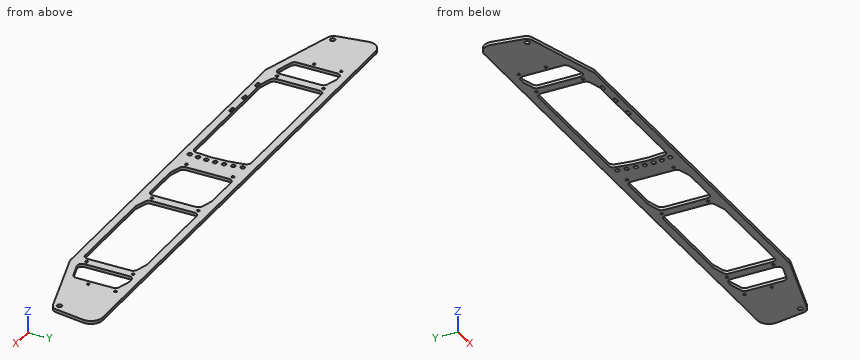
from build123d import *

# Parameters (mm, degrees)
SKETCH_1_R          = 3.25
EXTRUDE_1_DEPTH     = 4
HOLE_WIZARD_M52_D   = 5.5
HOLE_WIZARD_M53_D   = 5.5
FILLET_5_R          = 10
CUT_EXTRUDE_4_DEPTH = 354.032576401
FILLET_7_R          = 6
HOLE_WIZARD_M34_D   = 3.4
CUT_EXTRUDE_5_DEPTH = 354.032576401


with BuildPart() as part:
    # Эскиз1 → Бобышка-Вытянуть1 (new body)
    with BuildSketch(Plane.XY):
        with BuildLine():
            Line((-349.818316726, 28.672449915), (-342.910885265, -15.303620822))
            Line((-342.910885265, -15.303620822), (-240, -46))
            Line((-240, -46), (240, -46))
            Line((240, -46), (342.910885265, -15.303620822))
            Line((342.910885265, -15.303620822), (349.818316726, 28.672449915))
            ThreePointArc((349.818316726, 28.672449915), (346.399852001, 40.749019149), (335, 46))
            Line((335, 46), (-335, 46))
            ThreePointArc((-335, 46), (-346.399852001, 40.749019149), (-349.818316726, 28.672449915))
        make_face()
        with Locations((-335, -9.635315981)):
            Circle(SKETCH_1_R, mode=Mode.SUBTRACT)
        with Locations(Location((335, -9.635315981, 0), (0, 0, 180))):
            Circle(SKETCH_1_R, mode=Mode.SUBTRACT)
    extrude(amount=EXTRUDE_1_DEPTH)

    # Отверстие с зазором M52 (through all)
    with Locations(Plane(origin=(0, 0, 0), x_dir=(-1, 0, 0), z_dir=(0, 0, -1))):
        with Locations((215, -7)):
            Hole(HOLE_WIZARD_M52_D / 2)

    # Отверстие с зазором M53 (through all)
    with Locations(Plane(origin=(0, 0, 0), x_dir=(-1, 0, 0), z_dir=(0, 0, -1))):
        with Locations((31.771314746, 9.83), (35.189476411, 32.040691677), (33.141482074, 20.990703059), (31.085819286, -1.380913569), (31.085819286, -12.619086431), (31.771893326, -23.836297834), (33.141482074, -34.990703059)):
            Hole(HOLE_WIZARD_M53_D / 2)

    # Скругление5
    fillet_5_edges = [part.edges().sort_by_distance(p)[0] for p in [
        (342.910885265, -15.303620822, 2),
        (240, -46, 2),
        (-240, -46, 2),
        (-342.910885265, -15.303620822, 2),
    ]]
    fillet(fillet_5_edges, radius=FILLET_5_R)

    # Эскиз22 → Вырез-Вытянуть4 (cut, through all)
    with BuildSketch(Plane(origin=(0, 0, 0), x_dir=(-1, 0, 0), z_dir=(0, 0, -1))):
        Polygon((-227.540368898, -36), (-98.70593747, -36), (-79.540368898, -30.283271798), (-79.540368898, 36), (-208.374800326, 36), (-227.540368898, 30.283271798), align=None)
        with BuildLine():
            Line((227.54, -30.283271798), (208.374431428, -36))
            Line((208.374431428, -36), (40.898736363, -36))
            ThreePointArc((40.898736363, -36), (38.644905491, 0.150569256), (43.818079226, 36))
            Line((43.818079226, 36), (227.54, 36))
            Line((227.54, 36), (227.54, -30.283271798))
        make_face()
        Polygon((-271, 30.283271798), (-251.834431428, 36), (-239.540368898, 36), (-239.540368898, -35.701718831), (-271, -26.317903284), align=None)
        Polygon((-67.540368898, -36), (-13.70593747, -36), (5.459631102, -30.283271798), (5.459631102, 36), (-48.374800326, 36), (-67.540368898, 30.283271798), align=None)
        Polygon((239.54, 30.283271798), (258.705568572, 36), (271, 36), (271, -26.317903284), (239.54, -35.701828866), align=None)
    extrude(amount=-CUT_EXTRUDE_4_DEPTH, mode=Mode.SUBTRACT)

    # Скругление7
    fillet_7_edges = [part.edges().sort_by_distance(p)[0] for p in [
        (227.540368898, -36, 2),
        (227.540368898, 30.283271798, 2),
        (208.374800326, 36, 2),
        (79.540368898, 36, 2),
        (79.540368898, -30.283271798, 2),
        (98.70593747, -36, 2),
        (271, -26.317903284, 2),
        (271, 30.283271798, 2),
        (251.834431428, 36, 2),
        (239.540368898, 36, 2),
        (239.540368898, -35.701718831, 2),
        (-40.898736363, -36, 2),
        (-43.818079226, 36, 2),
        (-227.54, 36, 2),
        (-227.54, -30.283271798, 2),
        (-208.374431428, -36, 2),
        (67.540368898, -36, 2),
        (67.540368898, 30.283271798, 2),
        (48.374800326, 36, 2),
        (-5.459631102, 36, 2),
        (-5.459631102, -30.283271798, 2),
        (13.70593747, -36, 2),
        (-271, -26.317903284, 2),
        (-239.54, -35.701828866, 2),
        (-239.54, 30.283271798, 2),
        (-258.705568572, 36, 2),
        (-271, 36, 2),
    ]]
    fillet(fillet_7_edges, radius=FILLET_7_R)

    # Отверстие с зазором M34 (through all)
    with Locations(Plane(origin=(0, 0, 0), x_dir=(-1, 0, 0), z_dir=(0, 0, -1))):
        with Locations((-233.540368898, 32), (-233.540368898, -28), (-73.540368898, -28), (-73.540368898, 32), (11.459631102, 32), (11.459631102, -28), (277, 32), (277, -3), (-277, 32), (-277, -3), (233.54, -28), (233.54, 32)):
            Hole(HOLE_WIZARD_M34_D / 2)

    # Эскиз25 → Вырез-Вытянуть5 (cut, through all)
    with BuildSketch(Plane.XY.offset(4)):
        with BuildLine():
            Line((-208.641482074, -37.3), (-203.641482074, -37.3))
            ThreePointArc((-203.641482074, -37.3), (-201.941482074, -39), (-203.641482074, -40.7))
            Line((-203.641482074, -40.7), (-208.641482074, -40.7))
            ThreePointArc((-208.641482074, -40.7), (-210.341482074, -39), (-208.641482074, -37.3))
        make_face()
        with BuildLine():
            Line((-177.141482074, -37.3), (-172.141482074, -37.3))
            ThreePointArc((-172.141482074, -37.3), (-170.441482074, -39), (-172.141482074, -40.7))
            Line((-172.141482074, -40.7), (-177.141482074, -40.7))
            ThreePointArc((-177.141482074, -40.7), (-178.841482074, -39), (-177.141482074, -37.3))
        make_face()
        with BuildLine():
            Line((-140.641482074, -40.7), (-145.641482074, -40.7))
            ThreePointArc((-145.641482074, -40.7), (-147.341482074, -39), (-145.641482074, -37.3))
            Line((-145.641482074, -37.3), (-140.641482074, -37.3))
            ThreePointArc((-140.641482074, -37.3), (-138.941482074, -39), (-140.641482074, -40.7))
        make_face()
    extrude(amount=-CUT_EXTRUDE_5_DEPTH, mode=Mode.SUBTRACT)


solid = part.part
Work out the finished part from the listing and answer in its coordinate system (mm). Round coordinates to 2 decimals unless told otherwise and drop trailing zeros. Write each loop counter-clockwise with the first axis right and the second up, starting at its lowest first coordinate (ties: lowest second). Pieces come first, ordered by that corner, then holes.
1) Straight lines are drawn through the part: line 1 (Y direction, x = -233.54, z = 2); line 2 (Y direction, x = -206, z = 2.1); line 3 (Y direction, x = 102.5, z = 2.9). For each, find the intervals that lie inside material, in ascending order.
2) Given pin 1 Ø1.2 at (y, z) = (11, 2) entering from +X, flat-ended and moving along its own axis, determine where the tip first touches the part or whether it passes through.
3) A cutting plane is placed at D-D (x = -294). Give the vertices of the cut face in (y, z), plus the area to 3 significant figures.
4) A cutting plane is placed at A-A (x = -164.5). Give the vertices of the cut face in (y, z), plus the area to 3 significant figures.
5) A cutting plane is placed at C-C (x = 260). Give the vertices of the cut face in (y, z).
6) A cutting plane is placed at B-B (z = 3.35). Give the number of separate pieces and of enclosed holes in the cut face, plus the area to 3 significant figures.
Completed:
1. line 1: y = -46 to -29.7, -26.3 to 30.3, 33.7 to 46
1. line 2: y = -46 to -40.7, -37.3 to -36, 36 to 46
1. line 3: y = -46 to -36, 36 to 46
2. pin 1: stops at x = 347.14
3. outline: (-29.89, 0) - (46, 0) - (46, 4) - (-29.89, 4) - close
3. area: 304 mm2
4. outline: (-46, 0) - (-36, 0) - (-36, 4) - (-46, 4) - close; (36, 0) - (46, 0) - (46, 4) - (36, 4) - close
4. area: 80.0 mm2
5. outline: (-40.03, 0) - (-29.6, 0) - (-29.6, 4) - (-40.03, 4) - close; (33.56, 0) - (46, 0) - (46, 4) - (33.56, 4) - close
6. separate pieces: 1
6. enclosed holes: 29
6. area: 26,800 mm2
